```python
from build123d import *

# Parameters (mm, degrees)
SKETCH1_R                = 50
BOSS_EXTRUDE1_DEPTH      = 20
BOSS_EXTRUDE2_DEPTH      = 52
BOSS_EXTRUDE2_DEPTH_BACK = 82
SKETCH2_R                = 4
SKETCH3_R                = 4
SKETCH3_R_2              = 3.5
CUT_EXTRUDE1_DEPTH       = 1


with BuildPart() as part:
    # Sketch1 → Boss-Extrude1 (new, symmetric)
    with BuildSketch(Plane.XY):
        Circle(SKETCH1_R)
    extrude(amount=BOSS_EXTRUDE1_DEPTH, both=True)

    # Sketch2 → Boss-Extrude2 (add, two sides: drawn at the far end of the back side and taken through both)
    with BuildSketch(Plane.XY.offset(20).offset(-BOSS_EXTRUDE2_DEPTH_BACK)):
        Circle(SKETCH2_R)
    extrude(amount=BOSS_EXTRUDE2_DEPTH + BOSS_EXTRUDE2_DEPTH_BACK)

    # Sketch3 → Cut-Extrude1 (cut)
    with BuildSketch(Plane(origin=(0, 0, -50), x_dir=(-1, 0, 0), z_dir=(0, 0, -1))):
        with Locations(Location((0, 0, 0), (0, 0, 180))):
            Circle(SKETCH3_R)
        Circle(SKETCH3_R_2, mode=Mode.SUBTRACT)
    cut_extrude1 = extrude(amount=-CUT_EXTRUDE1_DEPTH, mode=Mode.SUBTRACT)

    # Mirror1: Cut-Extrude1 across plane
    add(cut_extrude1.mirror(Plane.XY), mode=Mode.SUBTRACT)


solid = part.part
```
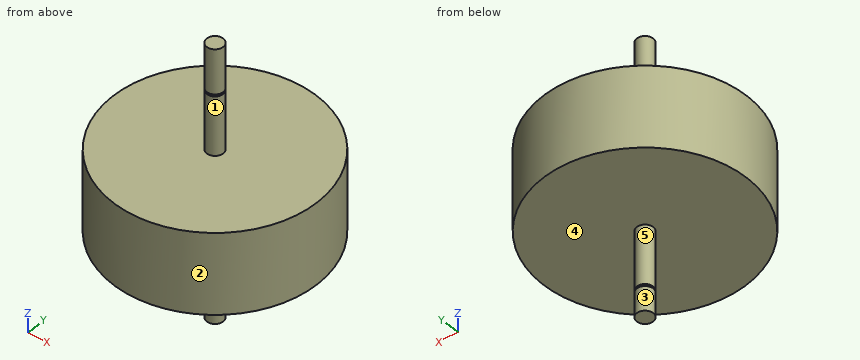
Work out the finished part from the listing and answer in its coordinate system (mm). Face numbers are marked on the shaded views. A direction names the side the tool comes from. Coordinates: 2 decimals unless noted, no trailing zeros. Loops run counter-clockwise (first coordinate to the right, second up) from the corner with the lowest first, then second, coordinate; pieces in that order, holes last. Notation, with made-up numbers: (-20.5, 9.5) -> (-16.5, 9.5) arc R26 cw to (-16.5, 26.5) -> close; hole circle Ø7 at (-33, -5.75). An arc over 180 degrees is marked (long way). Answer as CSV lines item,"result".
Q1. A tool of negligible diameter and unlimited length cuts with its end or side. For the marked faces 1, 2 and 3, from which of +Z, -Z, +X, -X, +Y, -Y can it reach the whole face along a straight path? Write none if from no direction.
Findings:
face 1,"+Z"
face 2,"+Z, -Z"
face 3,"-Z"
Q2. The part is cut by section A-A on y = 0. Write down the section's boundary in (x, z), and give its area (3 significant figures).
Findings:
outline,"(-50, -20) -> (-4, -20) -> (-4, -49) -> (-3.5, -49) -> (-3.5, -50) -> (-4, -50) -> (-4, -62) -> (4, -62) -> (4, -50) -> (3.5, -50) -> (3.5, -49) -> (4, -49) -> (4, -20) -> (50, -20) -> (50, 20) -> (4, 20) -> (4, 49) -> (3.5, 49) -> (3.5, 50) -> (4, 50) -> (4, 72) -> (-4, 72) -> (-4, 50) -> (-3.5, 50) -> (-3.5, 49) -> (-4, 49) -> (-4, 20) -> (-50, 20) -> close"
area,"4,750 mm²"
Q3. The part is cut by section C-C on z = -13.5. Write down the section's boundary in (x, y).
Findings:
outline,"circle Ø100 at (0, 0)"
Q4. Find the intervals of material crossed by probe 1 along Z at (x, y) = (-23.5, -20); probe 2 along X at (y, z) = (-10, 17); probe 3 along Y at (x, z) = (5, -17), in increasing order.
Findings:
probe 1,"z = -20 to 20"
probe 2,"x = -48.99 to 48.99"
probe 3,"y = -49.75 to 49.75"
Q5. Each of these flat-tipped pins is pushed along its axis until it touches: pin 1 (12 mm diameter, centred on x = -6.5, y = -39, fed in from +Z); pin 2 (10 mm diameter, centred on x = 31.5, z = 4, fed in from +Y); pin 3 (6 mm diameter, centred on y = -13, z = -15.5, fed in from -X). Where does it stop, or does it pass through?
Findings:
pin 1,"stops at z = 20"
pin 2,"stops at y = 42.4"
pin 3,"stops at x = -48.99"
Q6. For a pull along X with two mould halves and no side action, classify the marked faces 4 and 5 as +X half, -X half, draft (parallel to the pull), parting line (faces both ways), or undercut.
Findings:
face 4,"draft"
face 5,"parting line"
Q7. The part is cut by section D-D on z = 45.5. Write down the section's boundary in (x, y), and give its area (3 significant figures).
Findings:
outline,"circle Ø8 at (0, 0)"
area,"50.3 mm²"
